from build123d import *

# Parameters (mm, degrees)
SKETCH_1_R      = 2
SKETCH_1_R_2    = 1.25
EXTRUDE_1_DEPTH = 3
FILLET_1_R      = 1


with BuildPart() as part:
    # 草图1 → 凸台-拉伸1 (new body)
    with BuildSketch(Plane.XY):
        Polygon((10, 0), (10, 21), (5, 21), (5, 29), (10, 29), (0, 39), (0, 0), align=None)
        with Locations((5, 14)):
            Circle(SKETCH_1_R, mode=Mode.SUBTRACT)
        with Locations((2, 2)):
            Circle(SKETCH_1_R_2, mode=Mode.SUBTRACT)
        with Locations((8, 2)):
            Circle(SKETCH_1_R_2, mode=Mode.SUBTRACT)
    extrude(amount=EXTRUDE_1_DEPTH)

    # 圆角1
    fillet_1_edges = [part.edges().sort_by_distance(p)[0] for p in [
        (0, 39, 1.5),
        (10, 0, 1.5),
        (0, 0, 1.5),
    ]]
    fillet(fillet_1_edges, radius=FILLET_1_R)


solid = part.part
Read the model definition and answer for the solid it produces. Units are mm, in the model's axes. A direction names the side the tool comes from. Round coordinates to 2 decimals unless told otherwise and drop trailing zeros. Loops run counter-clockwise (first coordinate to the right, second up) from the corner with the lowest first, then second, coordinate; pieces in that order, holes last. Notation, with made-up numbers: (-12.5, -12.5) - (-4.5, -12.5) arc R13 ccw to (-4.5, 2.5) - close; hole circle Ø7 at (84.25, -6). An arc over 180 degrees is marked (long way). One line per question, with ' | ' between items. Start each with the question number.
Q1. For a pull along X with two mould halves and no side action, classify faces 3 (the flat face through (5, 25, 1)), 4 (the cylindrical face through (3.19, 2.38, 1.48)), 5 (the cylindrical face through (0.602, 37.503, 1.521)), 6 (the cylindrical face through (6.75, 2.05, 1.48)) as +X half, -X half, draft (parallel to the pull), parting line (faces both ways), or undercut.
Q2. Section A-A on x = 8 is taken. Give the vertices of the cut face in (y, z).
Q3. Find the intervals of material crossed by L1, parallel to X at y = 2.5, z = 1.5; L2, parallel to X at y = 26, z = 1.3; L3, parallel to X at y = 32, z = 0.6, in increasing order.
Q4. Section B-B on z = 2.2 is taken. Give the vertices of the cut face in (x, y).
Q5. Section C-C on y = 2 is taken. Give the vertices of the cut face in (x, z), plus the area to 3 significant figures.
Q6. For faces 1 (the flat face through (4, 19, 0)), 2 (the flat face through (7, 29, 1)), determine the directions among +Z, -Z, +X, -X, +Y, -Y from which every point of the face is accessible in a straight line to the end or side of a thin tool.
Q7. Flat-ended cylindrical pins translate along their axes: pin 1 (0.9 mm diameter, centred on y = 25.5, z = 2, fed in from +X); pin 2 (2 mm diameter, centred on x = 2, y = 2, fed in from +Z); pin 3 (1 mm diameter, centred on x = 5.5, z = 1.5, fed in from +Y). Find the tip coordinate at first contact, or state that the pin passes through.
Q8. Section D-D on x = 4.5 is taken. Give the vertices of the cut face in (y, z).
Established:
1) face 3: +X half | face 4: undercut | face 5: parting line | face 6: undercut
2) outline: (0, 0) - (0.75, 0) - (0.75, 3) - (0, 3) - close; (3.25, 0) - (21, 0) - (21, 3) - (3.25, 3) - close; (29, 0) - (31, 0) - (31, 3) - (29, 3) - close
3) L1: 0 to 0.85, 3.15 to 6.85, 9.15 to 10 | L2: 0 to 5 | L3: 0 to 7
4) outline: (0, 1) arc R1 ccw to (1, 0) - (9, 0) arc R1 ccw to (10, 1) - (10, 21) - (5, 21) - (5, 29) - (10, 29) - (1.71, 37.29) arc R1 ccw to (0, 36.59) - close; hole circle Ø2.5 at (2, 2); hole circle Ø4 at (5, 14); hole circle Ø2.5 at (8, 2)
5) outline: (0, 0) - (0.75, 0) - (0.75, 3) - (0, 3) - close; (3.25, 0) - (6.75, 0) - (6.75, 3) - (3.25, 3) - close; (9.25, 0) - (10, 0) - (10, 3) - (9.25, 3) - close | area: 15.0 mm²
6) face 1: -Z, +X, -X, +Y, -Y | face 2: +Z, -Z, +X
7) pin 1: x = 5 | pin 2: through | pin 3: y = 34
8) outline: (0, 0) - (12.06, 0) - (12.06, 3) - (0, 3) - close; (15.94, 0) - (34.5, 0) - (34.5, 3) - (15.94, 3) - close
